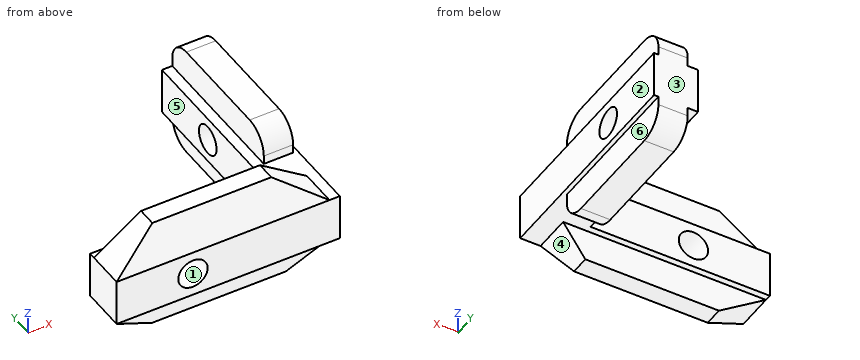
from build123d import *

# Parameters (mm, degrees)
EXTRUDE_1_DEPTH        = 4
EXTRUDE_1_DEPTH_BACK   = 4
EXTRUDE_2_DEPTH        = 36.25
CHAMFER_1_SIZE         = 8
CHAMFER_1_SIZE_2       = 5.5
EXTRUDE_3_DEPTH        = 2.5
EXTRUDE_3_DEPTH_BACK   = 2.5
HOLE_WIZARD_M6_1_D     = 5
HOLE_WIZARD_M6_1_DEPTH = 17
HOLE_WIZARD_M6_1_TIP   = 1.502151548
HOLE_WIZARD_M6_2_D     = 5
HOLE_WIZARD_M6_2_DEPTH = 17
HOLE_WIZARD_M6_2_TIP   = 1.502151548


with BuildPart() as part:
    # 草图1 → 凸台-拉伸1 (new, two sides: drawn at the far end of the back side and taken through both)
    with BuildSketch(Plane.XY.offset(-EXTRUDE_1_DEPTH_BACK)):
        Polygon((0, 7.5), (30.5, 7.5), (30.5, 38), (38, 38), (38, 0), (0, 0), align=None)
    extrude(amount=EXTRUDE_1_DEPTH + EXTRUDE_1_DEPTH_BACK)

    # 草图2 → 凸台-拉伸2 (add)
    with BuildSketch(Plane.ZY):
        Polygon((4, 6.4), (9.5, 6.4), (9.5, 3.2), (4, 0), align=None)
        Polygon((-4, 0), (-4, 6.4), (-9.5, 6.4), (-9.5, 3.2), align=None)
    extrude(amount=-EXTRUDE_2_DEPTH)

    # 倒角1
    # the kernel refuses this chamfer: 8, 5.5 mm, written as the material it takes off along each edge
    with BuildSketch(Plane(origin=(36.25, 27.064204354, -9.5), x_dir=(0.021932761143399794, 0, 0.9997594480616957), z_dir=(0, -1, 0))) as chamfer_1_piece_1_section:
        Polygon((CHAMFER_1_SIZE * 0.999759448062, CHAMFER_1_SIZE * 0.0219327611434), (-CHAMFER_1_SIZE_2 * 0.0219327611434, CHAMFER_1_SIZE_2 * 0.999759448062), (0, 0), align=None)
    chamfer_1_piece_1 = extrude(amount=44.528408708, mode=Mode.PRIVATE)
    chamfer_1_piece_1 = split(chamfer_1_piece_1, bisect_by=Plane(origin=(34.285815681, 4.8, -4), z_dir=(0, 0, -1)), keep=Keep.TOP, mode=Mode.PRIVATE)
    add(chamfer_1_piece_1, mode=Mode.SUBTRACT)
    with BuildSketch(Plane(origin=(36.25, 27.064204354, 9.5), x_dir=(0.046364447759701236, 0, -0.9989245907394302), z_dir=(0, -1, 0))) as chamfer_1_piece_2_section:
        Polygon((CHAMFER_1_SIZE_2 * 0.998924590739, -CHAMFER_1_SIZE_2 * 0.0463644477597), (-CHAMFER_1_SIZE * 0.0463644477597, -CHAMFER_1_SIZE * 0.998924590739), (0, 0), align=None)
    chamfer_1_piece_2 = extrude(amount=44.528408708, mode=Mode.PRIVATE)
    chamfer_1_piece_2 = split(chamfer_1_piece_2, bisect_by=Plane(origin=(33.577095366, 4.8, 4), z_dir=(0, 0, 1)), keep=Keep.TOP, mode=Mode.PRIVATE)
    add(chamfer_1_piece_2, mode=Mode.SUBTRACT)
    with BuildSketch(Plane(origin=(0, 27.064204354, 9.5), x_dir=(-0.046364447759701714, 0, -0.9989245907394302), z_dir=(0, -1, 0))) as chamfer_1_piece_3:
        Polygon((CHAMFER_1_SIZE_2 * 0.998924590739, CHAMFER_1_SIZE_2 * 0.0463644477597), (-CHAMFER_1_SIZE * 0.0463644477597, CHAMFER_1_SIZE * 0.998924590739), (0, 0), align=None)
    extrude(amount=44.528408708, mode=Mode.SUBTRACT)
    with BuildSketch(Plane(origin=(0, 27.064204354, -9.5), x_dir=(-0.046364447759701714, 0, 0.9989245907394302), z_dir=(0, -1, 0))) as chamfer_1_piece_4:
        Polygon((CHAMFER_1_SIZE_2 * 0.998924590739, -CHAMFER_1_SIZE_2 * 0.0463644477597), (-CHAMFER_1_SIZE * 0.0463644477597, -CHAMFER_1_SIZE * 0.998924590739), (0, 0), align=None)
    extrude(amount=44.528408708, mode=Mode.SUBTRACT)

    # 草图3 → 凸台-拉伸3 (add, two sides: drawn at the far end of the back side and taken through both)
    with BuildSketch(Plane.ZY.offset(-34.75).offset(-EXTRUDE_3_DEPTH_BACK)):
        with BuildLine():
            Line((4, 38), (5.5, 38))
            ThreePointArc((5.5, 38), (8.328427125, 36.828427125), (9.5, 34))
            Line((9.5, 34), (9.5, 16))
            ThreePointArc((9.5, 16), (8.328427125, 13.171572875), (5.5, 12))
            Line((5.5, 12), (4, 12))
            Line((4, 12), (4, 38))
        make_face()
        with BuildLine():
            Line((-9.5, 34), (-9.5, 16))
            ThreePointArc((-9.5, 16), (-8.328427125, 13.171572875), (-5.5, 12))
            Line((-5.5, 12), (-4, 12))
            Line((-4, 12), (-4, 38))
            Line((-4, 38), (-5.5, 38))
            ThreePointArc((-5.5, 38), (-8.328427125, 36.828427125), (-9.5, 34))
        make_face()
    extrude(amount=EXTRUDE_3_DEPTH + EXTRUDE_3_DEPTH_BACK)

    # M6 螺纹孔1
    with Locations(Plane(origin=(30.5, 25, 0), x_dir=(0, 0, -1), z_dir=(-1, 0, 0))):
        with Locations((0, 0)):
            Hole(HOLE_WIZARD_M6_1_D / 2, depth=HOLE_WIZARD_M6_1_DEPTH)
            with Locations((0, 0, -(HOLE_WIZARD_M6_1_DEPTH + HOLE_WIZARD_M6_1_TIP / 2))):  # 118° drill point
                Cone(0, HOLE_WIZARD_M6_1_D / 2, HOLE_WIZARD_M6_1_TIP, mode=Mode.SUBTRACT)

    # M6 螺纹孔2
    with Locations(Plane(origin=(13, 7.5, 0), x_dir=(0, 0, 1), z_dir=(0, 1, 0))):
        with Locations((0, 0)):
            Hole(HOLE_WIZARD_M6_2_D / 2, depth=HOLE_WIZARD_M6_2_DEPTH)
            with Locations((0, 0, -(HOLE_WIZARD_M6_2_DEPTH + HOLE_WIZARD_M6_2_TIP / 2))):  # 118° drill point
                Cone(0, HOLE_WIZARD_M6_2_D / 2, HOLE_WIZARD_M6_2_TIP, mode=Mode.SUBTRACT)


solid = part.part
Read the model definition and answer for the solid it produces. Units are mm, in the model's axes. Face numbers are marked on the shaded views. A direction names the side the tool comes from. Coordinates: 2 decimals unless noted, no trailing zeros. Order: outer loops, then holes, each group sorted by start corner. A loop starts at its lowest first (then second) coordinate and runs counter-clockwise, first axis right, second up. Notation, with made-up numbers: (10, 62.25) -> (27, 62.25) arc R31 ccw to (27, 89.25) -> close; hole circle Ø5 at (87, 84). An arc over 180 degrees is marked (long way). Answer as a JSON object with one key per item and string values.
1) Consider line 1 along X through (y, z) = (2, 0); line 2 along Z through (x, y) = (32.5, 25); line 3 along Z through (x, y) = (32, 25). Determine where each line is inside the solid, lowest interval first. Write a range as from..to.
Model answer:
{"line 1": "x = 0..10.5, 15.5..38", "line 2": "z = -9.5..-2.5, 2.5..9.5", "line 3": "z = -4..-2.5, 2.5..4"}
2) The mould has two halves that part along X. Classify the marked faces 1, 2 and 3: released by +X, released by -X, zero draft, split by the parting line, or undercut.
Model answer:
{"face 1": "undercut", "face 2": "released by +X", "face 3": "zero draft"}
3) A cutting plane is placed at B-B, the plane y = 25. Determine the outline of the cut face in (x, z), plus the area to 3 significant figures.
Model answer:
{"outline": "(30.5, -4) -> (32.25, -4) -> (32.25, -9.5) -> (37.25, -9.5) -> (37.25, -4) -> (38, -4) -> (38, -2.5) -> (30.5, -2.5) -> close; (30.5, 2.5) -> (38, 2.5) -> (38, 4) -> (37.25, 4) -> (37.25, 9.5) -> (32.25, 9.5) -> (32.25, 4) -> (30.5, 4) -> close", "area": "77.5 mm²"}
4) Each of these flat-tipped pins is pushed along its axis until it touches: pin 1 (3 mm diameter, centred on y = 21, z = -6, fed in from -X); pin 2 (4.5 mm diameter, centred on x = 14, z = -8, fed in from +Y); pin 3 (2.5 mm diameter, centred on y = 26.5, z = -1.5, fed in from -X); pin 4 (2.5 mm diameter, centred on x = 13.5, z = -0.5, fed in from +Y). Where does it stop, or does it pass through?
Model answer:
{"pin 1": "stops at x = 32.25", "pin 2": "stops at y = 6.4", "pin 3": "stops at x = 30.5", "pin 4": "passes through"}
5) A cutting plane is placed at D-D, the plane y = 5.5. Determine the outline of the cut face in (x, z).
Model answer:
{"outline": "(0, -4) -> (8, -9.5) -> (30.75, -9.5) -> (34.53, -4) -> (38, -4) -> (38, 4) -> (36.25, 4) -> (28.25, 9.5) -> (8, 9.5) -> (0, 4) -> close; hole circle Ø5 at (13, 0)"}
6) A cutting plane is placed at A-A, the plane z = 0. Determine the outline of the cut face in (x, y), plus the area to 3 significant figures.
Model answer:
{"outline": "(0, 0) -> (10.5, 0) -> (10.5, 7.5) -> (0, 7.5) -> close; (15.5, 0) -> (38, 0) -> (38, 22.5) -> (30.5, 22.5) -> (30.5, 7.5) -> (15.5, 7.5) -> close; (30.5, 27.5) -> (38, 27.5) -> (38, 38) -> (30.5, 38) -> close", "area": "439 mm²"}
7) A tool of negligible diameter and unlimited length cuts with its end or side. For the marked faces 4, 5 and 6, from which of +Z, -Z, +X, -X, +Y, -Y can it reach the whole face along a straight path? Write none if from no direction.
Model answer:
{"face 4": "-Z, +X, -Y", "face 5": "+Z, -Z, -X, +Y", "face 6": "-Z, +X, +Y, -Y"}
8) A cutting plane is placed at C-C, the plane x = 13. Determine the outline of the cut face in (y, z).
Model answer:
{"outline": "(0, -4) -> (3.2, -9.5) -> (6.4, -9.5) -> (6.4, -4) -> (7.5, -4) -> (7.5, -2.5) -> (0, -2.5) -> close; (0, 2.5) -> (7.5, 2.5) -> (7.5, 4) -> (6.4, 4) -> (6.4, 9.5) -> (3.2, 9.5) -> (0, 4) -> close"}
